Part print with two shaded views. Sizes in mm from the minimum x, y, z corner. Round coordinates to 2 decimals unless told otherwise and drop trailing zeros. Loops run counter-clockwise (first coordinate to the right, second up) from the corner with the lowest first, then second, coordinate; pieces in that order, holes last. Notation, with made-up numbers: (11.25, 70.25) - (42.25, 70.25) arc R12 ccw to (42.25, 84.25) - close; hole circle Ø10 at (-5, -0.75). An arc over 180 degrees is marked (long way). Use a Markdown table: item, result.
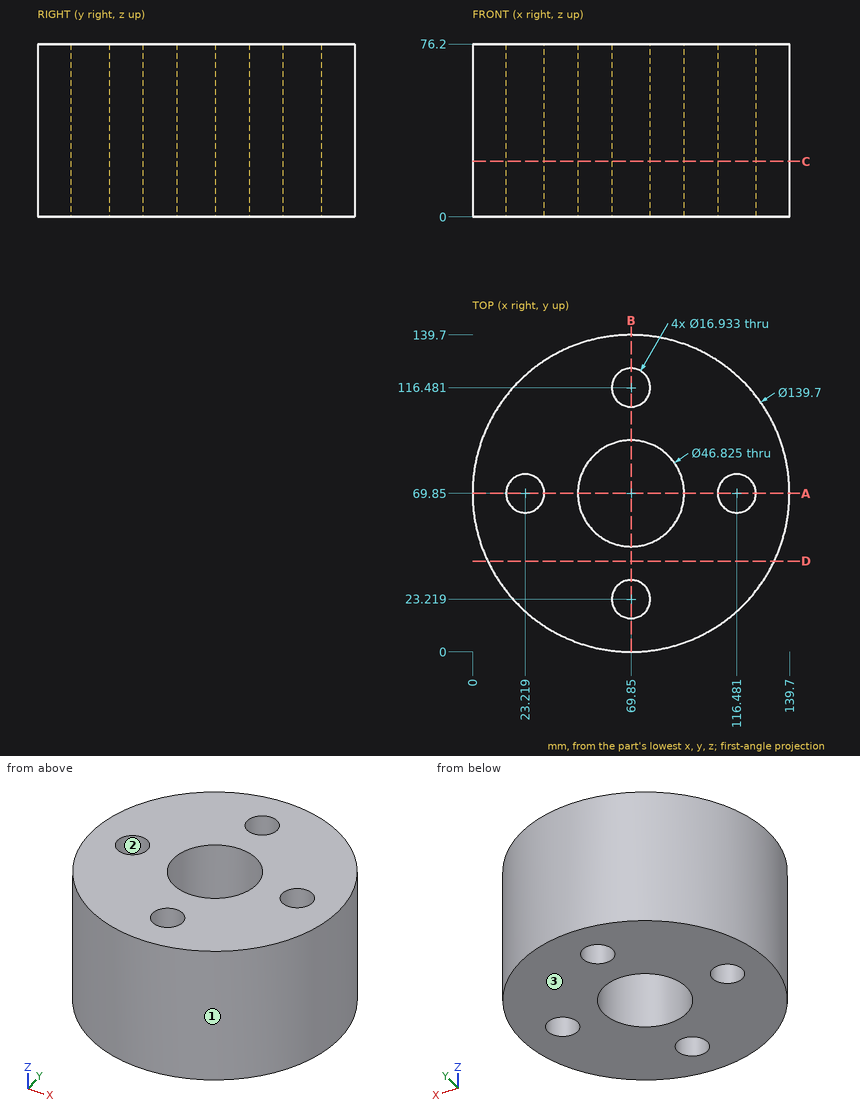
Q1. Cut at C-C, the plane z = 24.5. Count the separate pieces of the cut face and the enclosed holes in it, plus the area to 3 significant figures.
Results found:
| item | result |
|---|---|
| separate pieces | 1 |
| enclosed holes | 5 |
| area | 12,700 mm2 |
Q2. Probe line 1 (Y direction, x = 69.85, z = 32) (1 decimal); line 2 (Y direction, x = 65, z = 20) (1 decimal); line 3 (X direction, y = 75.5, z = 62) (1 decimal). List the from-to ranges inside material, lowest first.
Results found:
| item | result |
|---|---|
| line 1 | y = 0 to 14.8, 31.7 to 46.4, 93.3 to 108, 124.9 to 139.7 |
| line 2 | y = 0.2 to 16.3, 30.2 to 46.9, 92.8 to 109.5, 123.4 to 139.5 |
| line 3 | x = 0.2 to 16.9, 29.5 to 47.1, 92.6 to 110.2, 122.8 to 139.5 |
Q3. Drop flat-ended pins along their axis: pin 1 (3 mm diameter, centred on x = 92, z = 54, fed in from -Y); pin 2 (10 mm diameter, centred on x = 54, z = 8.5, fed in from +Y); pin 3 (3 mm diameter, centred on y = 68, z = 33, fed in from +X). Give the stop position or say it passes through.
Results found:
| item | result |
|---|---|
| pin 1 | stops at y = 3.12 |
| pin 2 | stops at y = 138.85 |
| pin 3 | stops at x = 139.7 |
Q4. Cut at D-D, the plane y = 40. List the corners of the cut face in (x, z).
Results found:
| item | result |
|---|---|
| outline | (6.7, 0) - (133, 0) - (133, 76.2) - (6.7, 76.2) - close |
Q5. Pull direction Y, two halves, no side cores. Call the marked faces 1, 2 and 3: pulls with the +Y half, pulls with the -Y half, needs draft (parallel to the pull), parting line crosses it, or undercut.
Results found:
| item | result |
|---|---|
| face 1 | parting line crosses it |
| face 2 | undercut |
| face 3 | needs draft |
Q6. Cut at A-A, the plane y = 69.85. List the corners of the cut face in (x, z) (1 decimal), plus the area to 3 significant figures.
Results found:
| item | result |
|---|---|
| outline | (0, 0) - (14.8, 0) - (14.8, 76.2) - (0, 76.2) - close; (31.7, 0) - (46.4, 0) - (46.4, 76.2) - (31.7, 76.2) - close; (93.3, 0) - (108, 0) - (108, 76.2) - (93.3, 76.2) - close; (124.9, 0) - (139.7, 0) - (139.7, 76.2) - (124.9, 76.2) - close |
| area | 4,500 mm2 |
